Autodesk Inventor part; units mm, degrees
ref_plane "YZ Plane" through (0, 0, 0) normal (1, 0, 0) x (0, 1, 0)
ref_plane "XZ Plane" through (0, 0, 0) normal (0, 1, 0) x (-1, 0, 0)
ref_plane "XY Plane" through (0, 0, 0) normal (0, 0, 1) x (1, 0, 0)
sketch "Sketch1" plane through (0, 0, 0) normal (0, 0, 1) x (1, 0, 0)
  line L0 (-20.4019, 15.1575) -> (4.9981, 15.1575)
  line L1 (4.9981, 15.1575) -> (4.9981, 6.2675)
  line L2 (4.9981, 6.2675) -> (-20.4019, 6.2675)
  line L3 (-20.4019, 6.2675) -> (-20.4019, 15.1575)
  arc A0 (0.5531, 6.2675) -> (0.5531, 15.1575) centre (0.5531, 10.7125) ccw
  circle A1 centre (-15.9569, 10.7125) radius 1.905
  circle A2 centre (0.5531, 10.7125) radius 1.905
  line L4 (-8.6544, 13.8875) -> (-6.7494, 13.8875)
  line L5 (-6.7494, 13.8875) -> (-6.7494, 7.5375)
  line L6 (-6.7494, 7.5375) -> (-8.6544, 7.5375)
  line L7 (-8.6544, 7.5375) -> (-8.6544, 13.8875)
  point P0 (0, 0)
  dimension "d0" = 25.4
  dimension "d1" = 8.89
  dimension "d2" = 0
  dimension "d3" = 0
  dimension "d4" = 3.81
  dimension "d5" = 3.81
  dimension "d6" = 0
  dimension "d7" = 4.445
  dimension "d8" = 4.445
  dimension "d9" = 7.3025
  dimension "d12" = 1.905
  dimension "d13" = 6.35
extrude "Extrusion1" add sketch "Sketch1" along normal blind 34.29 contours L0 A0 L2 L3
sketch "Sketch2" plane through (0, 0, 0) normal (0, 0, -1) x (-1, 0, 0)
  circle A0 centre (15.9569, 10.7125) radius 1.905
  circle A1 centre (15.9569, 10.7125) radius 1.905
  circle A2 centre (15.9569, 10.7125) radius 3.81
  point P0 (0, 0)
  dimension "d19" = 7.62
extrude "Extrusion2" add sketch "Sketch2" along normal blind 2.54 contours A0 | A2
sketch "Sketch3" plane through (-15.9569, 10.7125, -2.54) normal (0, 0, -1) x (-1, 0, 0)
  circle A0 centre (0, 0) radius 3.81
  circle A1 centre (0, 0) radius 3.175
  point P0 (-15.9569, -10.7125)
  dimension "d22" = 6.35
extrude "Extrusion3" add sketch "Sketch3" along normal blind 5.08 contours A1
sketch "Sketch4" plane through (-15.9569, 10.7125, -7.62) normal (0, 0, -1) x (-1, 0, 0)
  circle A0 centre (0, 0) radius 3.81
  circle A1 centre (0, 0) radius 3.81
  point P0 (-15.9569, -10.7125)
extrude "Extrusion4" add sketch "Sketch4" along normal blind 1.27
sketch "Sketch5" plane through (0, 0, 34.29) normal (0, 0, 1) x (1, 0, 0)
  arc A0 (0.5531, 6.2675) -> (0.5531, 15.1575) centre (0.5531, 10.7125) ccw
  circle A1 centre (0.5531, 10.7125) radius 2.54
  point P0 (0, 0)
  dimension "d27" = 5.08
extrude "Extrusion5" add sketch "Sketch5" along normal blind 1.27
sketch "Sketch6" plane through (0.5531, 10.7125, 35.56) normal (0, 0, 1) x (1, 0, 0)
  circle A0 centre (0, 0) radius 2.54
  line L0 (-0.635, 1.905) -> (0.635, 1.905)
  line L1 (0.635, 1.905) -> (0.635, -1.905)
  line L2 (0.635, -1.905) -> (-0.635, -1.905)
  line L3 (-0.635, -1.905) -> (-0.635, 1.905)
  point P0 (-0.5531, -10.7125)
  dimension "d30" = 3.81
  dimension "d31" = 1.27
  dimension "d32" = 0.635
  dimension "d33" = 1.905
extrude "Extrusion6" add sketch "Sketch6" along normal blind 5.08 contours L0 L1 L2 L3
properties part number "Vacuum Valve 1764"
For this review, take the finished solid that the model builds, in its own axes (mm). A direction names the side the tool comes from. Give positions to 0.01 mm unless a question says otherwise; leave off trailing zeros. Loops run counter-clockwise (first coordinate to the right, second up) from the corner with the lowest first, then second, coordinate; pieces in that order, holes last. Notation, with made-up numbers: M -9.75,-3.5 L 15.25,-3.5 A21 ccw 15.25,20.5 Z; hole C -25,-27.75 d10. An arc over 180 degrees is marked long. Put each result on its own line as item: value. Start each with the question number.
(1) Add section A-A, the plane z = 24. Write out the cut boundary in (x, y) (1 decimal), then the cut area to 3 significant figures.
(2) For pin 1 (1.1 mm diameter, centred on x = 1.5, y = 10.5, fed in from -Z); pin 2 (5 mm diameter, centred on y = 14, z = -3, fed in from -X); pin 3 (4 mm diameter, centred on y = 11.5, z = 39.5, fed in from -X), all flat-tipped, find the tip position at first contact; note any pin that passes through.
(3) The part is to be moulded in two halves that separate along Y. For faces 1 (the flat face through (-8.654, 11, 17)), 2 (the flat face through (1, 11, 34.29)), 3 (the cylindrical face through (0, 13.19, 34.92)), 4 (the flat face through (-15, 14, -2.54)), say which applies: +Y half, -Y half, draft (parallel to the pull), parting line (faces both ways), or undercut.
(4) Machinability: for faces 5 (the flat face through (1, 8.808, 38)), 6 (the cylindrical face through (0.14, 12.572, 16.905)), 7 (the flat face through (-6.749, 11, 17)), 8 (the flat face through (1.188, 11, 38)), 9 (the flat face through (-0.082, 11, 38)), which of the approach directions +Z, -Z, +X, -X, +Y, -Y give a long, thin tool a straight path to every point of the face, cutting with its end or side? Answer none if there is none.
(5) Add section B-B, the plane x = -2.75. Write out the cut boundary in (y, z).
(6) Add section D-D, the plane x = 1.75. Write out the cut boundary in (y, z).
(7) Wall thickness on L1, parallel to X at y = 10.75, z = 28; L2, parallel to Y at x = -8.5, z = 13; L3, parallel to X at y = 11, z = 33: over which ranges is each line inside the solid? List them lowest first.
Result:
1. outline: M -20.4,6.3 L 0.6,6.3 A4.4 ccw 0.6,15.2 L -20.4,15.2 Z; hole C -16,10.7 d3.8; hole M -8.7,7.5 L -6.7,7.5 L -6.7,13.9 L -8.7,13.9 Z; hole C 0.6,10.7 d3.8
1. area: 182 mm^2
2. pin 1: stops at z = 34.29
2. pin 2: stops at x = -19.68
2. pin 3: stops at x = -0.08
3. face 1: undercut
3. face 2: undercut
3. face 3: parting line
3. face 4: draft
4. face 5: +Z, +X, -X, -Y
4. face 6: -Z
4. face 7: +Z, -Z
4. face 8: +Z, +X, +Y, -Y
4. face 9: +Z, -X, +Y, -Y
5. outline: M 6.27,0 L 15.16,0 L 15.16,34.29 L 6.27,34.29 Z
6. outline: M 6.43,0 L 9.23,0 L 9.23,34.29 L 12.19,34.29 L 12.19,0 L 14.99,0 L 14.99,34.29 L 12.95,34.29 L 12.95,35.56 L 8.47,35.56 L 8.47,34.29 L 6.43,34.29 Z
7. L1: x = -20.4 to -17.86, -14.05 to -8.65, -6.75 to -1.35, 2.46 to 5
7. L2: y = 6.27 to 7.54, 13.89 to 15.16
7. L3: x = -20.4 to -17.84, -14.07 to -8.65, -6.75 to -1.33, 2.44 to 4.99
